from build123d import *

# Parameters (mm, degrees)
ESQUISSE1_R        = 1.25
ESQUISSE1_R_2      = 1.5
BOSS_EXTRU_1_DEPTH = 3
CONG_3_R           = 22
CONG_4_R           = 22


with BuildPart() as part:
    # Esquisse1 → Boss.-Extru.1 (new body)
    with BuildSketch(Plane.XY):
        with BuildLine():
            Line((-8.227794557, 2.434117026), (4.272205443, 2.434117026))
            Line((4.272205443, 2.434117026), (4.272205443, -12.832640321))
            add(Edge.make_bspline(
                [(-8.227794557, -12.832640321), (-1.977794557, -32.832640321), (4.272205443, -12.832640321)],
                knots=[0, 0, 0, 1, 1, 1], degree=2))
            Line((-8.227794557, -12.832640321), (-8.227794557, 2.434117026))
        make_face()
        with Locations((-4.977794557, -2.832640321)):
            Circle(ESQUISSE1_R, mode=Mode.SUBTRACT)
        with Locations((1.022205443, -2.832640321)):
            Circle(ESQUISSE1_R, mode=Mode.SUBTRACT)
        with Locations((-1.977794557, -12.832640321)):
            Circle(ESQUISSE1_R_2, mode=Mode.SUBTRACT)
    extrude(amount=BOSS_EXTRU_1_DEPTH)

    # Congé3
    cong_3_edges = [part.edges().sort_by_distance(p)[0] for p in [
        (4.272205443, -12.832640321, 1.5),
    ]]
    fillet(cong_3_edges, radius=CONG_3_R)

    # Congé4
    cong_4_edges = [part.edges().sort_by_distance(p)[0] for p in [
        (-8.227794557, -12.832640321, 1.5),
    ]]
    fillet(cong_4_edges, radius=CONG_4_R)


solid = part.part
Can you work these out from the model? Positions are in its coordinate system, mm. Coordinates: 2 decimals unless noted, no trailing zeros. Loops run counter-clockwise (first coordinate to the right, second up) from the corner with the lowest first, then second, coordinate; pieces in that order, holes last. Notation, with made-up numbers: M 86,87.25 L 108,87.25 A24 ccw 108,113.25 Z; hole C -21.5,-2 d10. An arc over 180 degrees is marked long. Return JSON: item names as keys, results as strings. Group by question number.
Item 1: Imagine slicing it at B-B (z = 0.25). Give the number of separate pieces and of enclosed holes in the cut face, and give its area (3 significant figures).
Item 2: Imagine slicing it at A-A (y = -2). Please give me the cut outline in (x, z), and give its area (3 significant figures).
Item 3: I'm going to push flat-ended pins straight in: pin 1 Ø1 at (x, z) = (1, 2.5) entering from -Y; pin 2 Ø1 at (y, z) = (-13, 0.5) entering from -X. Where does each tip first touch, or does it pass through?
Item 4: If I drill on L1, parallel to X at y = -3.75, z = 0.5; L2, parallel to Y at x = -5.25, z = 0.35; L3, parallel to Y at x = 0, z = 1.9, over which ranges is the centre line in solid material (lowest first)? Write a range as from..to.
Verdict:
{
 "1": {"separate pieces": "1", "enclosed holes": "3", "area": "255 mm^2"},
 "2": {"outline": "M -8.23,0 L -5.91,0 L -5.91,3 L -8.23,3 Z; M -4.05,0 L 0.09,0 L 0.09,3 L -4.05,3 Z; M 1.95,0 L 4.27,0 L 4.27,3 L 1.95,3 Z", "area": "26.3 mm^2"},
 "3": {"pin 1": "stops at y = -21.26", "pin 2": "stops at x = -7.95"},
 "4": {"L1": "x = -8.23..-5.83, -4.13..0.17, 1.87..4.27", "L2": "y = -20.09..-4.05, -1.61..2.43", "L3": "y = -21.83..-3.55, -2.11..2.43"}
}
